The drawing under review shows one solid part. Ordinate dimensions are in mm from its lowest x, y, z. A direction names the side the tool comes from. Coordinates: 2 decimals unless noted, no trailing zeros. Loops run counter-clockwise (first coordinate to the right, second up) from the corner with the lowest first, then second, coordinate; pieces in that order, holes last. Notation, with made-up numbers: M 70.25,32 L 125.25,32 A28 ccw 125.25,52 Z; hole C 46,-7 d10. An arc over 180 degrees is marked long. Return JSON: item names as keys, results as strings.
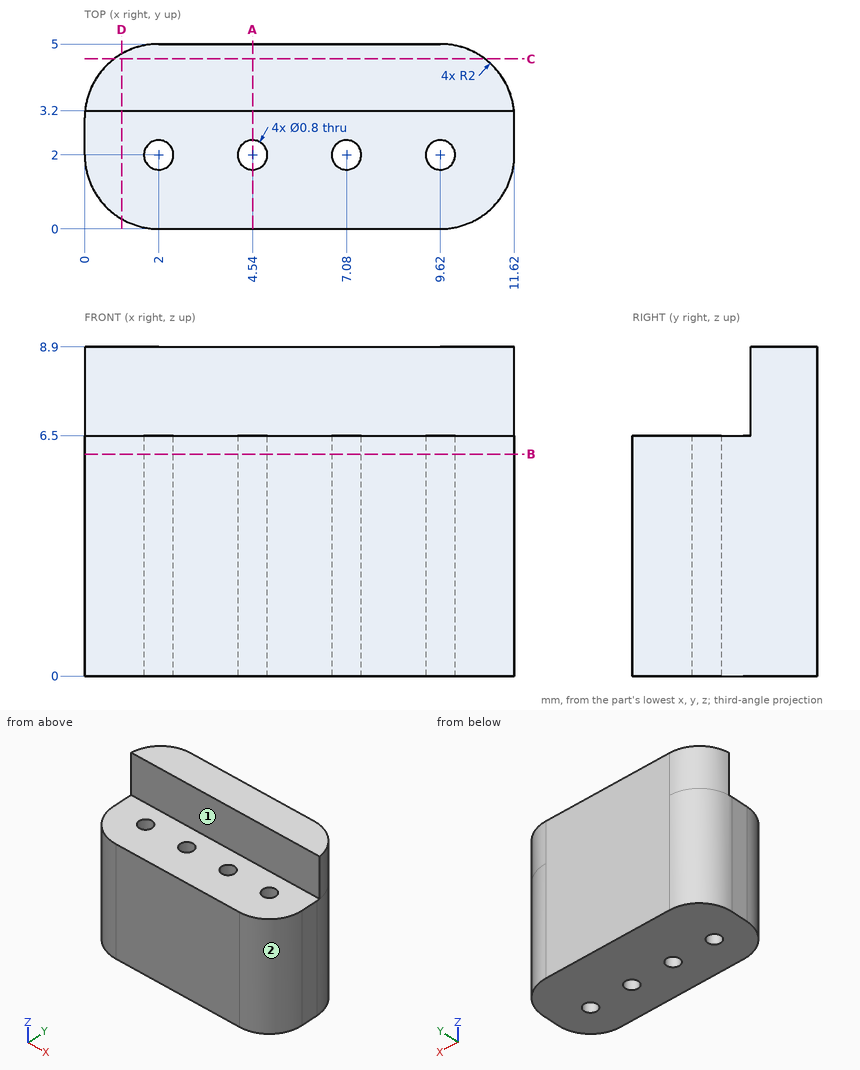
1. Add section C-C on y = 4.6. Give the boundary of the cut face in (x, z).
Check values:
{"outline": "M 0.8,0 L 10.82,0 L 10.82,8.9 L 0.8,8.9 Z"}
2. Insertion check: pin 1 Ø1.5 at (y, z) = (2, 7.5) entering from -X; pin 2 Ø0.7 at (x, z) = (8, 8) entering from -Y. Each pin has a flat end and moves straight along its axis. Give the tip position at first contact, or say it passes through.
Check values:
{"pin 1": "through", "pin 2": "y = 3.2"}
3. Add section A-A on x = 4.54. Give the boundary of the cut face in (y, z), plus the area to 3 significant figures.
Check values:
{"outline": "M 0,0 L 1.6,0 L 1.6,6.5 L 0,6.5 Z; M 2.4,0 L 5,0 L 5,8.9 L 3.2,8.9 L 3.2,6.5 L 2.4,6.5 Z", "area": "31.6 mm²"}
4. Machinability: for the marked faces 1 and 2, which of the approach directions +Z, -Z, +X, -X, +Y, -Y give a long, thin tool a straight path to every point of the face, cutting with its end or side? Answer none if there is none.
Check values:
{"face 1": "+Z, +X, -X, -Y", "face 2": "+Z, -Z, +X, -Y"}
5. Add section B-B on z = 6. Give the boundary of the cut face in (x, y), plus the area to 3 significant figures.
Check values:
{"outline": "M 0,2 A2 ccw 2,0 L 9.62,0 A2 ccw 11.62,2 L 11.62,3 A2 ccw 9.62,5 L 2,5 A2 ccw 0,3 Z; hole C 2,2 d0.8; hole C 4.54,2 d0.8; hole C 7.08,2 d0.8; hole C 9.62,2 d0.8", "area": "52.7 mm²"}
6. To check wall thickness, follow line 1 (Y direction, x = 7.08, z = 4); line 2 (Z direction, x = 8.5, y = 1.25); line 3 (Y direction, x = 4.25, z = 8.5). State the ranges of each line that lie inside material, in increasing order.
Check values:
{"line 1": "0 to 1.6, 2.4 to 5", "line 2": "0 to 6.5", "line 3": "3.2 to 5"}
7. Add section D-D on x = 1. Give the boundary of the cut face in (y, z), plus the area to 3 significant figures.
Check values:
{"outline": "M 0.27,0 L 4.73,0 L 4.73,8.9 L 3.2,8.9 L 3.2,6.5 L 0.27,6.5 Z", "area": "32.7 mm²"}
